Read the model definition and answer for the solid it produces. Units are mm, in the model's axes. A direction names the side the tool comes from. Give positions to 0.01 mm unless a question says otherwise; leave off trailing zeros. Order: outer loops, then holes, each group sorted by start corner. A loop starts at its lowest first (then second) coordinate and runs counter-clockwise, first axis right, second up. Notation, with made-up numbers: (62.5, -0.5) - (74.5, -0.5) arc R10 ccw to (74.5, 9.5) - close; hole circle Ø11 at (-38.5, 69.5). An arc over 180 degrees is marked (long way). Answer as CSV lines item,"result". Start each with the question number.
from build123d import *

# Parameters (mm, degrees)
F0_R     = 2.25
F1_DEPTH = 15


with BuildPart() as f1:
    # F0 (on Top) → F1 (new body)
    with BuildSketch(Plane.XY):
        with BuildLine():
            Line((31.366729, -182.725793), (34.111926, -185.285689))
            ThreePointArc((34.111926, -185.285689), (35.991225, -183.270417), (38.043709, -181.431833))
            Line((38.043709, -181.431833), (35.117688, -178.703318))
            ThreePointArc((35.117688, -178.703318), (35.764119, -179.617985), (35.992209, -180.714555))
            ThreePointArc((35.992209, -180.714555), (34.338779, -183.236466), (31.366729, -182.725793))
        make_face()
        with BuildLine():
            Line((27.097168, -200.814555), (27.097168, -226.214555))
            Line((27.097168, -226.214555), (47.097168, -226.214555))
            Line((47.097168, -226.214555), (47.097168, -221.914555))
            ThreePointArc((47.097168, -221.914555), (58.633169, -222.668244), (69.219767, -218.023751))
            ThreePointArc((69.219767, -218.023751), (71.312849, -216.22702), (73.189601, -214.205377))
            ThreePointArc((73.189601, -214.205377), (76.96026, -207.928201), (78.697168, -200.814555))
            ThreePointArc((78.697168, -200.814555), (72.02437, -182.90062), (54.797168, -174.614555))
            ThreePointArc((54.797168, -174.614555), (45.906812, -176.760956), (38.043709, -181.431833))
            ThreePointArc((38.043709, -181.431833), (35.991225, -183.270417), (34.111926, -185.285689))
            ThreePointArc((34.111926, -185.285689), (29.505205, -192.553523), (27.097168, -200.814555))
        make_face()
        with BuildLine():
            ThreePointArc((35.117688, -178.703318), (31.230971, -178.839076), (31.366729, -182.725793))
            ThreePointArc((31.366729, -182.725793), (34.338779, -183.236466), (35.992209, -180.714555))
            ThreePointArc((35.992209, -180.714555), (35.764119, -179.617985), (35.117688, -178.703318))
        make_face()
        with Locations((33.242209, -180.714555)):
            Circle(F0_R, mode=Mode.SUBTRACT)
        with BuildLine():
            ThreePointArc((73.189601, -214.205377), (71.312849, -216.22702), (69.219767, -218.023751))
            Line((69.219767, -218.023751), (72.921689, -221.475793))
            ThreePointArc((72.921689, -221.475793), (72.785931, -217.589076), (76.672648, -217.453318))
            Line((76.672648, -217.453318), (73.189601, -214.205377))
        make_face()
        with BuildLine():
            ThreePointArc((76.672648, -217.453318), (72.785931, -217.589076), (72.921689, -221.475793))
            ThreePointArc((72.921689, -221.475793), (75.893738, -221.986466), (77.547168, -219.464555))
            ThreePointArc((77.547168, -219.464555), (77.319079, -218.367985), (76.672648, -217.453318))
        make_face()
        with Locations((74.797168, -219.464555)):
            Circle(F0_R, mode=Mode.SUBTRACT)
    extrude(amount=-F1_DEPTH)


solid = f1.part
(1) Flat-ended cylindrical pins translate along their axes: pin 1 Ø4 at (x, y) = (74.8, -219.46) entering from -Z; pin 2 Ø6 at (x, z) = (55, -10.5) entering from -Y; pin 3 Ø2 at (x, z) = (68, -7) entering from +Y; pin 4 Ø4 at (x, z) = (66, -8.5) entering from -Y. Find the tip coordinate at first contact, or state that the pin passes through.
(2) Section A-A, the plane x = 75 is taken. Write down the section's boundary in (y, z), and give its area (3 significant figures).
(3) Straight lines are drawn through the part: line 1 (X direction, y = -179.5, z = -9.5); line 2 (X direction, y = -182, z = -14); line 3 (Y direction, x = 35, z = -8.25). For each, find the intervals that lie inside material, in ascending order. Write a range as [from, to].
(4) Which of the six approach directions +Z, -Z, +X, -X, +Y, -Y give full straight-line access (tool end or side, diameter ignored) to faces 1 (the cylindrical face through (31.27, -178.8, -7.4)), 2 (the flat face through (32.72, -183.99, -7.4)), 3 (the cylindrical face through (46.03, -176.71, -7.4)), 4 (the flat face through (47.097, -224, -7)), 5 (the flat face through (74.956, -215.852, -7.395))?
(5) Section B-B, the plane z = -7.5 is taken. Write down the section's boundary in (x, y), and give its area (3 significant figures).
(6) Determine the mould class of faces 6 (the cylindrical face through (73.01, -220.83, -7.4)), 7 (the flat face through (53, -200, 0)), 8 (the flat face through (71.045, -219.726, -7.395)) for opening direction Y: released by +Y, released by -Y, zero draft, split by the parting line, or undercut.
(7) Section C-C, the plane y = -195 is taken. Write down the section's boundary in (x, z).
(8) Section D-D, the plane x = 44 is taken. Write down the section's boundary in (y, z), and give its area (3 significant figures).
Checks:
1,pin 1,"passes through"
1,pin 2,"stops at y = -223.04"
1,pin 3,"stops at y = -178.65"
1,pin 4,"stops at y = -221.07"
2,outline,"(-222.21, -15) - (-221.71, -15) - (-221.71, 0) - (-222.21, 0) - close; (-217.22, -15) - (-215.89, -15) - (-215.89, 0) - (-217.22, 0) - close; (-211.71, -15) - (-186.88, -15) - (-186.88, 0) - (-211.71, 0) - close"
2,area,"400 mm²"
3,line 1,"x = [30.77, 31.35], [35.14, 35.97], [40.68, 68.24]"
3,line 2,"x = [30.81, 31.4], [35.09, 71.16]"
3,line 3,"y = [-226.21, -182.12], [-179.31, -178.6]"
4,face 1,"+Z, -Z"
4,face 2,"+Z, -Z, -X"
4,face 3,"+Z, -Z, +Y"
4,face 4,"+Z, -Z, -Y"
4,face 5,"+Z, -Z, +X"
5,outline,"(27.1, -226.21) - (47.1, -226.21) - (47.1, -221.91) arc R24.38 ccw to (69.22, -218.02) - (72.92, -221.48) arc R2.75 ccw to (77.55, -219.46) arc R2.75 ccw to (76.67, -217.45) - (73.19, -214.21) arc R24.38 ccw to (78.7, -200.81) arc R25.58 ccw to (54.8, -174.61) arc R30.69 ccw to (38.04, -181.43) - (35.12, -178.7) arc R2.75 ccw to (31.37, -182.73) - (34.11, -185.29) arc R30.69 ccw to (27.1, -200.81) - close; hole circle Ø4.5 at (33.24, -180.71); hole circle Ø4.5 at (74.8, -219.46)"
5,area,"2,140 mm²"
6,face 6,"undercut"
6,face 7,"zero draft"
6,face 8,"released by -Y"
7,outline,"(28.52, -15) - (78.18, -15) - (78.18, 0) - (28.52, 0) - close"
8,outline,"(-226.21, -15) - (-177.61, -15) - (-177.61, 0) - (-226.21, 0) - close"
8,area,"729 mm²"
